from build123d import *

# Parameters (mm, degrees)
SKETCH_1_W             = 100
SKETCH_1_H             = 40
EXTRUDE_1_DEPTH        = 22
HOLE_WIZARD_M121_D     = 10.2
HOLE_WIZARD_M121_DEPTH = 26.75
HOLE_WIZARD_M121_TIP   = 3.064389157
SKETCH_5_R             = 9
CUT_EXTRUDE_1_DEPTH    = 7
FILLET_1_R             = 20


with BuildPart() as part:
    # Эскиз1 → Бобышка-Вытянуть1 (new body)
    with BuildSketch(Plane(origin=(0, 0, 0), x_dir=(1, 0, 0), z_dir=(0, 1, 0))):
        Rectangle(SKETCH_1_W, SKETCH_1_H)
    extrude(amount=EXTRUDE_1_DEPTH)

    # Отверстие обработанное метчиком M121
    with Locations(Plane(origin=(-30, 22, 0), x_dir=(0, 0, 1), z_dir=(0, 1, 0))):
        with Locations((0, 0), (0, 60)):
            Hole(HOLE_WIZARD_M121_D / 2, depth=HOLE_WIZARD_M121_DEPTH)
            with Locations((0, 0, -(HOLE_WIZARD_M121_DEPTH + HOLE_WIZARD_M121_TIP / 2))):  # 118° drill point
                Cone(0, HOLE_WIZARD_M121_D / 2, HOLE_WIZARD_M121_TIP, mode=Mode.SUBTRACT)

    # Эскиз5 → Вырез-Вытянуть1 (cut)
    with BuildSketch(Plane(origin=(0, 22, 0), x_dir=(1, 0, 0), z_dir=(0, 1, 0))):
        with Locations(Location((30, 0, 0), (0, 0, 270))):
            Circle(SKETCH_5_R)
        with Locations(Location((-30, 0, 0), (0, 0, 270))):
            Circle(SKETCH_5_R)
    extrude(amount=-CUT_EXTRUDE_1_DEPTH, mode=Mode.SUBTRACT)

    # Скругление1
    fillet_1_edges = [part.edges().sort_by_distance(p)[0] for p in [
        (50, 11, 20),
        (50, 11, -20),
        (-50, 11, -20),
        (-50, 11, 20),
    ]]
    fillet(fillet_1_edges, radius=FILLET_1_R - 0.0001)  # a hair under: the kernel refuses the full size


solid = part.part
Check sheet for the modelled part. Datum: model origin and axes. Units: mm. A direction names the side the tool comes from. Give positions to 0.01 mm unless a question says otherwise; leave off trailing zeros. Write each loop counter-clockwise with the first axis right and the second up, starting at its lowest first coordinate (ties: lowest second). Pieces come first, ordered by that corner, then holes. Notation, with made-up numbers: (77, 0) -> (88, 0) arc R28 ccw to (88, 24) -> close; hole circle Ø10 at (71.5, 76.5). An arc over 180 degrees is marked (long way). One line per item, written item: value. Start each with the question number.
Item 1: Section check A-A on y = 2.75. State how many separate pieces and enclosed holes the cut face has, then the cut area to 3 significant figures.
Item 2: Material ranges on probe 1 along X at (y, z) = (18.25, 0); probe 2 along X at (y, z) = (6.5, 0); probe 3 along Z at (x, y) = (27, 10), recorded low to high. Write a range as from..to.
Item 3: Draft check along Z on faces 1 (the cylindrical face through (43.986, 11.154, 14.297)), 2 (the cylindrical face through (-21.077, 18.549, -1.172)), 3 (the flat face through (0, 11, -20)), 4 (the cylindrical face through (37.59, 18.55, 4.84)). Enter one of: +Z half, -Z half, draft (parallel to the pull), parting line (faces both ways), or undercut.
Item 4: Section check C-C on x = 37. Record the cut outline in (y, z), then the cut area to 3 significant figures.
Item 5: Gauge pin test, flat ends, axial feed: pin 1 (4 mm diameter, centred on x = -32.5, y = 4.5, fed in from -Z); pin 2 (16 mm diameter, centred on x = -30, z = 0, fed in from +Y); pin 3 (9 mm diameter, centred on x = 30, z = 0, fed in from -Y); pin 4 (2 mm diameter, centred on y = 9.5, z = -3.5, fed in from -X). Record the tip position at first contact, or that the pin passes through.
Item 6: Section check B-B on z = 2. Record the cut outline in (x, y), then the cut area to 3 significant figures.
Item 7: Tool access check on faces 5 (the cylindrical face through (-34.5, 7.4, -2.4)), 6 (the flat face through (-34, 15, 4)). Record the directions out of +Z, -Z, +X, -X, +Y, -Y that give a thin tool (end or side, any length) a straight path to the whole face; none if there is none.
Item 8: Section check D-D on z = -14.5. Record the cut outline in (x, y), then the cut area to 3 significant figures.
Results list:
1. separate pieces: 1
1. enclosed holes: 2
1. area: 3,490 mm²
2. probe 1: -50..-39, -21..21, 39..50
2. probe 2: -50..-35.1, -24.9..24.9, 35.1..50
2. probe 3: -20..-4.12, 4.12..20
3. face 1: +Z half
3. face 2: undercut
3. face 3: -Z half
3. face 4: undercut
4. outline: (0, -18.74) -> (22, -18.74) -> (22, -5.66) -> (15, -5.66) -> (15, 5.66) -> (22, 5.66) -> (22, 18.74) -> (0, 18.74) -> close
4. area: 745 mm²
5. pin 1: z = -19.99
5. pin 2: y = 15
5. pin 3: through
5. pin 4: x = -49.84
6. outline: (-49.9, 0) -> (-34.69, 0) -> (-34.69, 15) -> (-38.77, 15) -> (-38.77, 22) -> (-49.9, 22) -> close; (-25.31, 0) -> (25.31, 0) -> (25.31, 15) -> (21.23, 15) -> (21.23, 22) -> (-21.23, 22) -> (-21.23, 15) -> (-25.31, 15) -> close; (34.69, 0) -> (49.9, 0) -> (49.9, 22) -> (38.77, 22) -> (38.77, 15) -> (34.69, 15) -> close
6. area: 1,670 mm²
7. face 5: +Y, -Y
7. face 6: +Y
8. outline: (-43.78, 0) -> (43.78, 0) -> (43.78, 22) -> (-43.78, 22) -> close
8. area: 1,930 mm²
